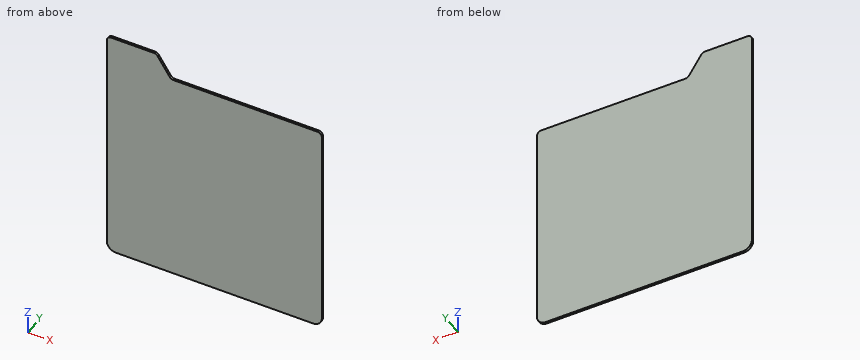
from build123d import *

# Parameters (mm, degrees)
F1_DEPTH = 1.5875
F2_R     = 6.35
F3_R     = 12.7


with BuildPart() as f1:
    # F0 (on Front) → F1 (new body, symmetric)
    with BuildSketch(Plane.XZ):
        Polygon((-152.4, 152.4), (-152.4, -152.4), (152.4, -152.4), (152.4, 152.4), (-61.4666454494, 152.4), (-82.55, 184.15), (-152.4, 184.15), align=None)
    extrude(amount=F1_DEPTH, both=True)

    # F2
    f2_edges = [f1.edges().sort_by_distance(p)[0] for p in [
        (152.4, 0, 152.4),
        (-152.4, 0, 184.15),
        (-61.466645, 0, 152.4),
        (-82.55, 0, 184.15),
    ]]
    fillet(f2_edges, radius=F2_R)

    # F3
    f3_edges = [f1.edges().sort_by_distance(p)[0] for p in [
        (152.4, 0, -152.4),
        (-152.4, 0, -152.4),
    ]]
    fillet(f3_edges, radius=F3_R)


solid = f1.part
The model under review builds one solid part; all positions refer to its coordinate system, in mm. Coordinates: 2 decimals unless noted, no trailing zeros. Write each loop counter-clockwise with the first axis right and the second up, starting at its lowest first coordinate (ties: lowest second). Pieces come first, ordered by that corner, then holes. Notation, with made-up numbers: (35.25, -33.5) - (81.25, -33.5) arc R14 ccw to (81.25, -15.5) - close; hole circle Ø3 at (14, 6.25). An arc over 180 degrees is marked (long way). Answer as a JSON object with one key per item and string values. Group by question number.
1. To check wall thickness, follow probe 1 along Z at (x, y) = (114, 0.6); probe 2 along X at (y, z) = (-1.1, 154); probe 3 along Z at (x, y) = (-76, 0.5). State the ranges of each line that lie inside material, in increasing order.
2. Clearance check with a flat-ended pin moving along its axis: pin 1 Ø1.5 at (x, y) = (-79.5, 0.5) entering from +Z. State where the tip first meets the part, or that it passes through.
3. Add section B-B (x = 110). Give the boundary of the cut face in (y, z).
4. Add section C-C (z = 160.5). Give the boundary of the cut face in (x, y), plus the area to 3 significant figures.
5. Add section A-A (y = -0.2). Give the boundary of the cut face in (x, z), plus the area to 3 significant figures.
Findings:
{
 "1": {"probe 1": "-152.4 to 152.4", "probe 2": "-152.4 to -62.28", "probe 3": "-152.4 to 174.29"},
 "2": {"pin 1": "z = 180.69"},
 "3": {"outline": "(-1.59, -152.4) - (1.59, -152.4) - (1.59, 152.4) - (-1.59, 152.4) - close"},
 "4": {"outline": "(-152.4, -1.59) - (-66.85, -1.59) - (-66.85, 1.59) - (-152.4, 1.59) - close", "area": "272 mm²"},
 "5": {"outline": "(-152.4, -139.7) arc R12.7 ccw to (-139.7, -152.4) - (139.7, -152.4) arc R12.7 ccw to (152.4, -139.7) - (152.4, 146.05) arc R6.35 ccw to (146.05, 152.4) - (-58.06, 152.4) arc R6.35 cw to (-63.35, 155.24) - (-80.67, 181.31) arc R6.35 ccw to (-85.96, 184.15) - (-146.05, 184.15) arc R6.35 ccw to (-152.4, 177.8) - close", "area": "95,400 mm²"}
}
